Autodesk Fusion 360 part; units mm, degrees
sketch "Sketch1" plane through (0, 0, 0) normal (0, 1, 0) x (1, 0, 0)
  circle A0 centre (0.0008, 24.9355) radius 3
  line L0 (2.5556, 32.9383) -> (-2.4444, 32.9383)
  line L1 (2.5556, 20.6375) -> (2.5556, -15.7025)
  line L2 (8, 25) -> (8, -20)
  circle A1 centre (0, -20) radius 3
  line L3 (-2.6799, 20.7149) -> (-2.6799, -15.7789)
  arc A2 (2.5556, 20.6375) -> (-2.6799, 20.7149) centre (0.0008, 24.9355) ccw
  arc A3 (-2.6799, -15.7789) -> (2.5556, -15.7025) centre (0, -20) ccw
  dimension "d1" = 6
  dimension "d2" = 10
  dimension "d4" = 5
  dimension "d5" = 36.34
  dimension "d6" = 45
  dimension "d7" = 6
sketch "Sketch2" plane through (0, 0, 0) normal (0, 1, 0) x (1, 0, 0)
  circle A0 centre (160, 0) radius 3
  line L0 (165.3043, -12.1067) -> (165.3043, 17.8933)
  line L1 (165.3043, -12.1067) -> (144.0787, -27.9224)
  line L2 (144.0787, -27.9224) -> (124.0787, -27.9224)
  line L3 (124.0787, -27.9224) -> (105.4535, -9.1138)
  line L4 (105.4535, -9.1138) -> (98.3535, -9.1138)
  line L5 (98.3535, -9.1138) -> (98.3535, 10.8862)
  line L6 (98.3535, 10.8862) -> (112.5535, 10.8862)
  line L7 (112.5535, 10.8862) -> (128, 34)
  line L8 (128, 34) -> (153, 34)
  line L9 (153, 34) -> (165.3043, 17.8933)
  circle A1 centre (144.0787, -15.0238) radius 3
  circle A2 centre (124.0787, -15.0238) radius 3
  line L10 (112.4283, -2.9974) -> (127.553, -3)
  line L11 (127.2855, 2.988) -> (112.556, 3)
  arc A3 (127.553, -3) -> (127.2855, 2.988) centre (127.5535, 0) ccw
  arc A4 (112.556, 3) -> (112.6778, -2.9974) centre (112.5535, 0) ccw
  circle A5 centre (128, 28) radius 2
  circle A6 centre (153, 28) radius 2
  dimension "d10" = 6
  dimension "d11" = 30
  dimension "d12" = 26.47
  dimension "d13" = 20
  dimension "d14" = 26.47
  dimension "d15" = 7.1
  dimension "d16" = 20
  dimension "d17" = 14.2
  dimension "d18" = 27.8
  dimension "d19" = 25
  dimension "d21" = 6
  dimension "d22" = 6
  dimension "d23" = 6
  dimension "d24" = 15
  dimension "d25" = 6
  dimension "d26" = 4
  dimension "d27" = 4
sketch "Sketch3" plane through (0, 0, 0) normal (0, 1, 0) x (1, 0, 0)
sketch "Sketch4" plane through (0, 0, 0) normal (0, 1, 0) x (1, 0, 0)
sketch "Sketch5" plane through (0, 0, 0) normal (0, 1, 0) x (1, 0, 0)
  circle A0 centre (0, -75) radius 3
  circle A1 centre (-0.0243, -126.973) radius 3
  line L0 (-20, -70) -> (-20, -141.97)
  line L1 (-5, -75) -> (-5, -112.8223)
  line L2 (5, -75) -> (5, -112.8395)
  arc A2 (5, -75) -> (-5, -75) centre (0, -75) ccw
  line L3 (-0.05, -141.973) -> (-0.05, -143.513)
  line L4 (-0.05, -143.513) -> (-0.4621, -143.739)
  line L5 (-0.4621, -143.739) -> (-1.4621, -143.739)
  line L6 (-1.4621, -143.739) -> (-1.9628, -143.2357)
  line L7 (-1.9628, -143.2357) -> (-1.9628, -141.8472)
  line L8 (-0.05, -145.0973) -> (-0.05, -123.9731)
  line L9 (-8.7204, -112.6318) -> (-7.8791, -112.0912)
  line L10 (-8.9448, -113.0448) -> (-8.7204, -112.6318)
  line L11 (-8.1122, -114.3403) -> (-8.9448, -113.0448)
  line L12 (-7.1857, -112.2439) -> (-6.4351, -113.412)
  line L13 (-7.8791, -112.0912) -> (-7.1857, -112.2439)
  line L14 (-12.4085, -115.6627) -> (-11.7536, -114.907)
  line L15 (-12.5075, -116.1222) -> (-12.4085, -115.6627)
  line L16 (-11.3436, -117.1306) -> (-12.5075, -116.1222)
  line L17 (-11.0453, -114.8581) -> (-9.996, -115.7674)
  line L18 (-11.7536, -114.907) -> (-11.0453, -114.8581)
  line L19 (-15.0933, -119.6099) -> (-14.6779, -118.7003)
  line L20 (-15.0589, -120.0786) -> (-15.0933, -119.6099)
  line L21 (-13.658, -120.7184) -> (-15.0589, -120.0786)
  line L22 (-14.012, -118.4539) -> (-12.749, -119.0307)
  line L23 (-14.6779, -118.7003) -> (-14.012, -118.4539)
  line L24 (-16.5573, -124.1536) -> (-16.415, -123.1638)
  line L25 (-16.3922, -124.5936) -> (-16.5573, -124.1536)
  line L26 (-14.8679, -124.8128) -> (-16.3922, -124.5936)
  line L27 (-15.8455, -122.7398) -> (-14.4712, -122.9374)
  line L28 (-16.415, -123.1638) -> (-15.8455, -122.7398)
  line L29 (-16.682, -128.9257) -> (-16.8243, -127.9359)
  line L30 (-16.3995, -129.3014) -> (-16.682, -128.9257)
  line L31 (-14.8752, -129.0822) -> (-16.3995, -129.3014)
  line L32 (-16.3973, -127.3686) -> (-15.023, -127.171)
  line L33 (-16.8243, -127.9359) -> (-16.3973, -127.3686)
  line L34 (-15.4571, -133.5396) -> (-15.8725, -132.63)
  line L35 (-15.0802, -133.8205) -> (-15.4571, -133.5396)
  line L36 (-13.6794, -133.1808) -> (-15.0802, -133.8205)
  line L37 (-15.6226, -131.9654) -> (-14.3596, -131.3886)
  line L38 (-15.8725, -132.63) -> (-15.6226, -131.9654)
  line L39 (-12.9819, -137.6215) -> (-13.6367, -136.8658)
  line L40 (-12.5412, -137.7849) -> (-12.9819, -137.6215)
  line L41 (-11.3773, -136.7764) -> (-12.5412, -137.7849)
  line L42 (-13.5843, -136.1577) -> (-12.5349, -135.2485)
  line L43 (-13.6367, -136.8658) -> (-13.5843, -136.1577)
  line L44 (-9.457, -140.8408) -> (-10.2982, -140.3002)
  line L45 (-8.9881, -140.8734) -> (-9.457, -140.8408)
  line L46 (-8.1555, -139.5779) -> (-8.9881, -140.8734)
  line L47 (-10.4473, -139.606) -> (-9.6967, -138.4379)
  line L48 (-10.2982, -140.3002) -> (-10.4473, -139.606)
  line L49 (-5.1679, -142.9365) -> (-6.1274, -142.6548)
  line L50 (-4.7088, -142.8357) -> (-5.1679, -142.9365)
  line L51 (-4.2749, -141.3581) -> (-4.7088, -142.8357)
  line L52 (-6.466, -142.0308) -> (-6.0748, -140.6985)
  line L53 (-6.1274, -142.6548) -> (-6.466, -142.0308)
  arc A3 (-5, -112.8223) -> (-6.4351, -113.412) centre (-0.0243, -126.973) ccw
  arc A4 (-8.1122, -114.3403) -> (-9.996, -115.7674) centre (-0.0243, -126.973) ccw
  arc A5 (-11.3436, -117.1306) -> (-12.749, -119.0307) centre (-0.0243, -126.973) ccw
  arc A6 (-13.658, -120.7184) -> (-14.4712, -122.9374) centre (-0.0243, -126.973) ccw
  arc A7 (-14.8679, -124.8128) -> (-15.023, -127.171) centre (-0.0243, -126.973) ccw
  arc A8 (-14.8752, -129.0822) -> (-14.3596, -131.3886) centre (-0.0243, -126.973) ccw
  arc A9 (-13.6794, -133.1808) -> (-12.5349, -135.2485) centre (-0.0243, -126.973) ccw
  arc A10 (-11.3773, -136.7764) -> (-9.6967, -138.4379) centre (-0.0243, -126.973) ccw
  arc A11 (-8.1555, -139.5779) -> (-6.0748, -140.6985) centre (-0.0243, -126.973) ccw
  arc A12 (-4.2749, -141.3581) -> (-1.9628, -141.8472) centre (-0.0243, -126.973) ccw
  arc A13 (-0.05, -141.973) -> (5, -112.8395) centre (-0.0243, -126.973) ccw
  dimension "d30" = 6
  dimension "d31" = 10
  dimension "d32" = 6
  dimension "d33" = 30
  dimension "d34" = 71.97
  dimension "d35" = 1.54
  dimension "d36" = 0.47
  dimension "d37" = 1
  dimension "d38" = 0.71
  dimension "d40" = 360
sketch "Sketch6" plane through (0, 0, 0) normal (0, 1, 0) x (1, 0, 0)
  circle A0 centre (135, -70) radius 3
  circle A1 centre (135, -95) radius 3
  line L0 (129.0014, -94.8707) -> (129, -70.0003)
  line L1 (141, -95) -> (141, -70)
  arc A2 (141, -70) -> (129, -70.0003) centre (135, -70) ccw
  line L2 (134.9353, -100.9997) -> (150.363, -126.7288)
  line L3 (138.9186, -99.5437) -> (196.6373, -196.6907)
  arc A3 (129.0014, -94.8707) -> (134.9353, -100.9997) centre (135, -95) ccw
  arc A4 (138.9186, -99.5437) -> (141, -95) centre (135, -95) ccw
  line L4 (196.6373, -196.6907) -> (189.4976, -203.5489)
  line L5 (189.4976, -203.5489) -> (182.5189, -204.0946)
  line L6 (179.3777, -201.8435) -> (142.738, -137.5509)
  arc A5 (179.3777, -201.8435) -> (182.5189, -204.0946) centre (182.2851, -201.1037) ccw
  arc A6 (142.2555, -135.5758) -> (142.738, -137.5509) centre (145.2387, -135.8936) ccw
  line L7 (150.363, -126.7288) -> (142.2555, -135.5758)
  dimension "d43" = 6
  dimension "d44" = 12
  dimension "d45" = 25
  dimension "d46" = 6
  dimension "d47" = 12
  dimension "d48" = 30
  dimension "d50" = 113
  dimension "d52" = 9.9
  dimension "d53" = 7
  dimension "d62" = 6
  dimension "d63" = 74
  dimension "d64" = 6
  dimension "d69" = 12
extrude "Extrude5" add sketch "Sketch6" along normal blind 10
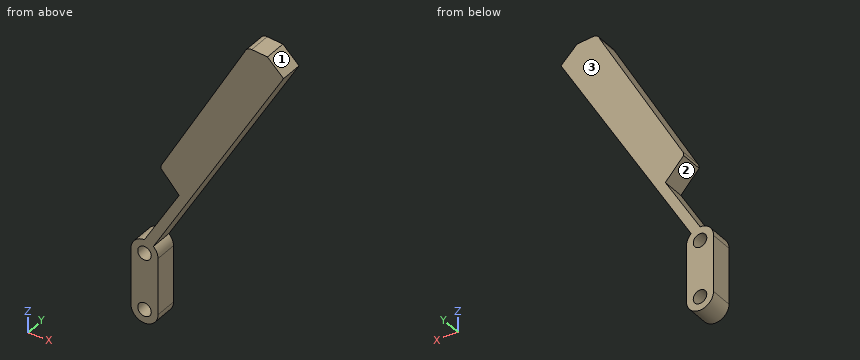
Source: CAD feature listing. Evaluate the final solid. Frame: model axes, mm. Face numbers are marked on the shaded views. Coordinates: 2 decimals unless noted, no trailing zeros. Order: outer loops, then holes, each group sorted by start corner. A loop starts at its lowest first (then second) coordinate and runs counter-clockwise, first axis right, second up. Notation, with made-up numbers: (-6.75, 87.5) - (38.25, 87.5) arc R29 ccw to (38.25, 117.5) - close; hole circle Ø5 at (17, 63). An arc over 180 degrees is marked (long way). One line per item, written item: value.
1) Mould query, pull axis Z, two halves, no side actions, for the marked faces 1, 2 and 3. Classes: released by +Z, released by -Z, zero draft, split by the parting line, or undercut.
Computed values:
face 1: released by +Z
face 2: undercut
face 3: zero draft
2) Cut plane A-A on y = 3. Output: boundary loops of the cut face in (x, z), plus the area to 3 significant figures.
Computed values:
outline: (129, 70) arc R6 ccw to (141, 70) - (141, 95) arc R6 ccw to (138.92, 99.54) - (196.64, 196.69) - (189.5, 203.55) - (182.52, 204.09) arc R3 ccw to (179.38, 201.84) - (142.74, 137.55) arc R3 ccw to (142.26, 135.58) - (150.36, 126.73) - (134.94, 101) arc R6 ccw to (129, 94.87) - close; hole circle Ø6 at (135, 70); hole circle Ø6 at (135, 95)
area: 1,870 mm^2
3) Cut plane C-C on x = 168. Output: boundary loops of the cut face in (y, z), plus the area to 3 significant figures.
Computed values:
outline: (0, 148.49) - (10, 148.49) - (10, 181.88) - (0, 181.88) - close
area: 334 mm^2
4) Contact query for flat-ended pins moving along their axis: pin 1 (5 mm diameter, centred on y = 5, z = 112.5, fed in from +X); pin 2 (3 mm diameter, centred on x = 139, y = 7, fed in from +Z); pin 3 (3.5 mm diameter, centred on x = 135, z = 70, fed in from +Y) (3 decimals); pin 4 (5 mm diameter, centred on y = 7, z = 84, fed in from +X). Output: stop coordinate, or through.
Computed values:
pin 1: stops at x = 148.1
pin 2: stops at z = 110.28
pin 3: passes through
pin 4: stops at x = 141
5) Ray query, line 1 (Z direction, x = 135, y = 8); line 2 (X direction, y = 3, z = 70); line 3 (Z direction, x = 135.5, y = 2.5). Return the intervals inside material, ascending. Write a range as [from, to].
Computed values:
line 1: z = [64, 67], [73, 92], [98, 101.11]
line 2: x = [129, 132], [138, 141]
line 3: z = [64.02, 67.04], [72.96, 92.04], [97.96, 101.94]
6) Cut plane B-B on z = 166.5. Output: boundary loops of the cut face in (x, y).
Computed values:
outline: (159.24, 0) - (178.7, 0) - (178.7, 10) - (159.24, 10) - close
